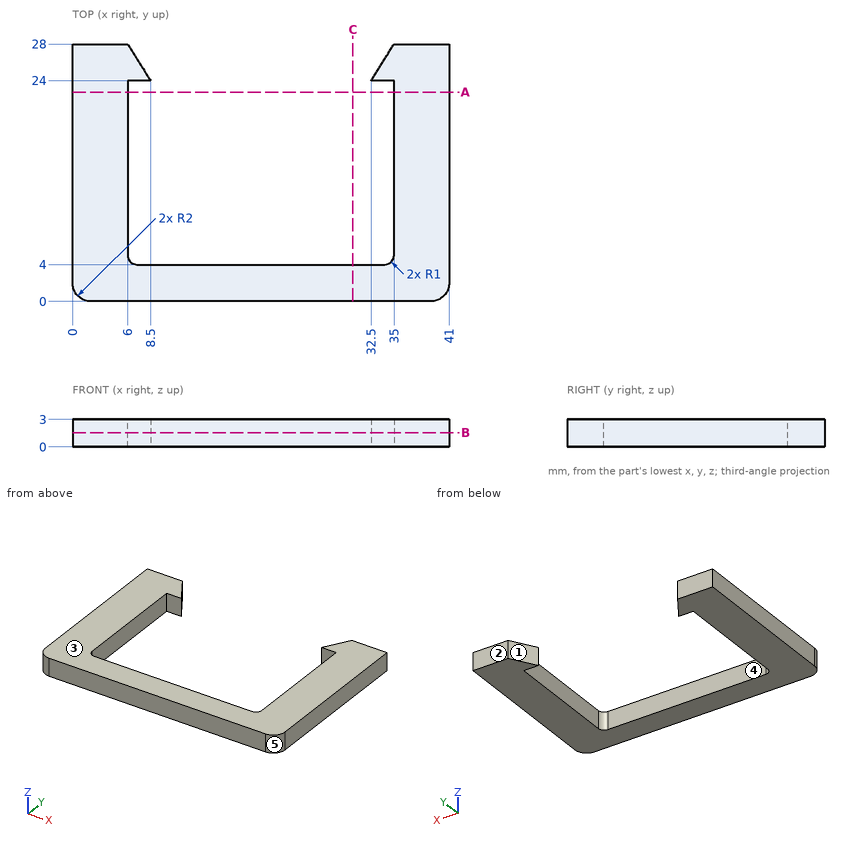
For this review, use the dimensioned drawing (mm, ordinates from the lowest corner) and the shaded views. A direction names the side the tool comes from. Round coordinates to 2 decimals unless told otherwise and drop trailing zeros. Order: outer loops, then holes, each group sorted by start corner. A loop starts at its lowest first (then second) coordinate and runs counter-clockwise, first axis right, second up. Notation, with made-up numbers: (-4.75, -29) -> (6.25, -29) arc R22 ccw to (6.25, -21) -> close; hole circle Ø9 at (-32, 27). An arc over 180 degrees is marked (long way). One line per item, written item: value. Start each with the question number.
Q1. Take a section at B-B (z = 1.55). Write out the cut boundary in (x, y).
Q2. Clearance check with flat-ended pins moving along their axes: pin 1 Ø12 at (x, y) = (15.5, 19.5) entering from +Z; pin 2 Ø1.5 at (x, z) = (19, 1.5) entering from +Y. State where each tip first meets the part, or that it passes through.
Q3. Take a section at A-A (y = 22.75). Write out the cut boundary in (x, z).
Q4. Take a section at C-C (x = 30.5). Write out the cut boundary in (y, z), and give its area (3 significant figures).
Q5. Wall thickness on line 1 (X direction, y = 19.5, z = 0.2); line 2 (Y direction, x = 14.5, z = 1.65); line 3 (Y direction, x = 34.5, z = 1.85): over which ranges is each line inside the solid? List them lowest first.
Q6. Machinability: for the marked faces 1 and 2, which of the approach directions +Z, -Z, +X, -X, +Y, -Y give a long, thin tool a straight path to every point of the face, cutting with its end or side? Answer none if there is none.
Q7. Mouldability with a two-part tool opening along X and no side actions: class the marked faces 3, 4 and 5 as released by +X, released by -X, zero draft, split by the parting line, or undercut.
Reported:
1. outline: (0, 2) arc R2 ccw to (2, 0) -> (39, 0) arc R2 ccw to (41, 2) -> (41, 28) -> (35, 28) -> (32.5, 24) -> (35, 24) -> (35, 5) arc R1 cw to (34, 4) -> (7, 4) arc R1 cw to (6, 5) -> (6, 24) -> (8.5, 24) -> (6, 28) -> (0, 28) -> close
2. pin 1: passes through
2. pin 2: stops at y = 4
3. outline: (0, 0) -> (6, 0) -> (6, 3) -> (0, 3) -> close; (35, 0) -> (41, 0) -> (41, 3) -> (35, 3) -> close
4. outline: (0, 0) -> (4, 0) -> (4, 3) -> (0, 3) -> close
4. area: 12.0 mm2
5. line 1: x = 0 to 6, 35 to 41
5. line 2: y = 0 to 4
5. line 3: y = 0 to 4.13, 24 to 27.2
6. face 1: +Z, -Z, +Y
6. face 2: +Z, -Z, +X, -X, +Y
7. face 3: zero draft
7. face 4: undercut
7. face 5: released by +X
